```python
from build123d import *

# Parameters (mm, degrees)
SKETCH1_W               = 40
SKETCH1_H               = 20.3
BOSS_EXTRUDE3_DEPTH     = 6
SHELL1_T                = -0.5
SKETCH4_W               = 7
SKETCH4_H               = 20.3
BOSS_EXTRUDE4_DEPTH     = 11
FILLET1_R               = 1
SKETCH5_R               = 2.1
SKETCH5_R_2             = 2.070075265
CUT_EXTRUDE3_DEPTH      = 6
SKETCH7_R               = 7
CUT_EXTRUDE4_DEPTH      = 88
CUT_EXTRUDE5_DEPTH      = 30.462221573
CUT_EXTRUDE5_DEPTH_BACK = 30.462221573
SKETCH8_R               = 2.1
SKETCH8_R_2             = 2.070075265


with BuildPart() as part:
    # Sketch1 → Boss-Extrude3 (new body)
    with BuildSketch(Plane(origin=(0, 0, 0), x_dir=(1, 0, 0), z_dir=(0, 1, 0))):
        Rectangle(SKETCH1_W, SKETCH1_H)
    extrude(amount=BOSS_EXTRUDE3_DEPTH)

    # Shell1
    shell1_openings = [part.faces().sort_by_distance(p)[0] for p in [
        (0, 0, 0),
    ]]
    offset(amount=SHELL1_T, openings=shell1_openings, kind=Kind.INTERSECTION)

    # Sketch4 → Boss-Extrude4 (add)
    with BuildSketch(Plane(origin=(0, 6, 0), x_dir=(1, 0, 0), z_dir=(0, 1, 0))):
        with Locations((-23.5, 0)):
            Rectangle(SKETCH4_W, SKETCH4_H)
        with Locations((23.5, 0)):
            Rectangle(SKETCH4_W, SKETCH4_H)
    extrude(amount=-BOSS_EXTRUDE4_DEPTH)

    # Fillet1
    fillet1_edges = [part.edges().sort_by_distance(p)[0] for p in [
        (-27, 0.5, 10.15),
        (-27, 0.5, -10.15),
        (27, 0.5, -10.15),
        (27, 0.5, 10.15),
    ]]
    fillet(fillet1_edges, radius=FILLET1_R)

    # Sketch5 → Cut-Extrude3 (cut)
    with BuildSketch(Plane.XZ.offset(5)):
        with Locations(Location((-24.35750849, 5.025, 0), (0, 0, 270))):
            Circle(SKETCH5_R)
        with Locations(Location((-24.35750849, -5.025, 0), (0, 0, 270))):
            Circle(SKETCH5_R)
        with Locations(Location((24.284171764, 5.025, 0), (0, 0, 270))):
            Circle(SKETCH5_R_2)
        with Locations(Location((24.284171764, -5.025, 0), (0, 0, 270))):
            Circle(SKETCH5_R)
    extrude(amount=-CUT_EXTRUDE3_DEPTH, mode=Mode.SUBTRACT)

    # Sketch7 → Cut-Extrude4 (cut)
    with BuildSketch(Plane.XZ.offset(-5.5)):
        with Locations(Location((-9.5, 0, 0), (0, 0, 270))):
            Circle(SKETCH7_R)
    extrude(amount=-CUT_EXTRUDE4_DEPTH, mode=Mode.SUBTRACT)

    # Sketch8 → Cut-Extrude5 (cut, two sides: drawn at the far end of the back side and taken through both)
    with BuildSketch(Plane.XZ.offset(-1).offset(-CUT_EXTRUDE5_DEPTH_BACK)):
        with Locations(Location((24.284171764, -5.025, 0), (0, 0, 270))):
            Circle(SKETCH8_R)
        with Locations(Location((24.284171764, 5.025, 0), (0, 0, 270))):
            Circle(SKETCH8_R_2)
        with Locations(Location((-24.35750849, 5.025, 0), (0, 0, 270))):
            Circle(SKETCH8_R)
        with Locations(Location((-24.35750849, -5.025, 0), (0, 0, 270))):
            Circle(SKETCH8_R)
    extrude(amount=CUT_EXTRUDE5_DEPTH + CUT_EXTRUDE5_DEPTH_BACK, mode=Mode.SUBTRACT)


solid = part.part
```
Could you check a few things on this model? Use its own coordinates, in mm. A direction names the side the tool comes from. Round coordinates to 2 decimals unless told otherwise and drop trailing zeros. Write each loop counter-clockwise with the first axis right and the second up, starting at its lowest first coordinate (ties: lowest second). Pieces come first, ordered by that corner, then holes. Notation, with made-up numbers: M 83,-12 L 110,-12 A19 cw 110,23 Z; hole C 13.25,71.25 d6. An arc over 180 degrees is marked long. Answer in a Markdown table with one row per item. Add a question column.
Q1. Imagine slicing it at B-B (z = 0). Please give me the cut outline in (x, y).
Q2. On a 3-axis mill with a long thin cutter (end or side, diameter ignored), from which of +Z, -Z, +X, -X, +Y, -Y can I reach the whole of each face in a straight line? I mean faces 5 (the flat face through (0, 0, -10)), 6 (the cylindrical face through (-26.221, 0.577, 4.056)), 7 (the flat face through (19.5, 3, 0)). Say none if no direction works.
Q3. Imagine slicing it at D-D (z = 4.5). Please give me the cut outline in (x, y).
Q4. Will this pin go through, and if not, where does the flat tip stop? pin 1 Ø6 at (x, z) = (0.5, -4.5) entering from -Y.
Q5. If I drill on line 1 (Z direction, x = 5, y = 2.25); line 2 (X direction, y = -1.75, z = 0.5); line 3 (X direction, y = 3, z = 1), over which ranges is the centre line in solid material (lowest first)? Write a range as from..to.
Q6. If we mould it in two halves opening along Z, with no side actions, what happens to faces 1 (the cylindrical face through (-26.715, 0.423, 9.849)), 2 (the cylindrical face through (-16.334, 5.746, 1.517)), 3 (the flat face through (0, 3, -9.65)), 4 (the flat face through (-24, -5, 0))? For each: +Z half, -Z half, draft (parallel to the pull), parting line (faces both ways), or undercut.
Q7. Imagine slicing it at A-A (y = -1.75). Give the number of separate pieces and of enclosed holes in the cut face, then the cut area to 3 significant figures.
Q8. Imagine slicing it at C-C (x = -9.5). Please give me the cut outline in (y, z), then the cut area to 3 significant figures.
Values:
| question | item | result |
|---|---|---|
| 1 | outline | M -27,-5 L -20,-5 L -20,0 L -19.5,0 L -19.5,5.5 L -16.5,5.5 L -16.5,6 L -27,6 Z; M -2.5,5.5 L 19.5,5.5 L 19.5,0 L 20,0 L 20,-5 L 27,-5 L 27,6 L -2.5,6 Z |
| 2 | face 5 | +Z, -Z, -Y |
| 2 | face 6 | +Y, -Y |
| 2 | face 7 | -Y |
| 3 | outline | M -27,-5 L -26.39,-5 L -26.39,6 L -27,6 Z; M -22.32,-5 L -20,-5 L -20,0 L -19.5,0 L -19.5,5.5 L -14.86,5.5 L -14.86,6 L -22.32,6 Z; M -4.14,5.5 L 19.5,5.5 L 19.5,0 L 20,0 L 20,-5 L 22.28,-5 L 22.28,6 L -4.14,6 Z; M 26.29,-5 L 27,-5 L 27,6 L 26.29,6 Z |
| 4 | pin 1 | y = 5.5 |
| 5 | line 1 | -10.15..-9.65, 9.65..10.15 |
| 5 | line 2 | -27..-20, 20..27 |
| 5 | line 3 | -27..-19.5, 19.5..27 |
| 6 | face 1 | +Z half |
| 6 | face 2 | undercut |
| 6 | face 3 | undercut |
| 6 | face 4 | draft |
| 7 | separate pieces | 2 |
| 7 | enclosed holes | 4 |
| 7 | area | 228 mm^2 |
| 8 | outline | M 0,-10.15 L 6,-10.15 L 6,-7 L 5.5,-7 L 5.5,-9.65 L 0,-9.65 Z; M 0,9.65 L 5.5,9.65 L 5.5,7 L 6,7 L 6,10.15 L 0,10.15 Z |
| 8 | area | 8.65 mm^2 |
